from build123d import *

# Parameters (mm, degrees)
F0_R     = 75
F1_DEPTH = 3.5
F2_R     = 1.6
F3_DEPTH = 3.5
F5_DEPTH = 3.5
F6_R     = 1.6
F7_DEPTH = 3.5
F8_W     = 1.85
F8_H     = 28.2
F9_DEPTH = 3.501


with BuildPart() as f1:
    # F0 (on Top) → F1 (new body)
    with BuildSketch(Plane.XY):
        Circle(F0_R)
    extrude(amount=F1_DEPTH)

    # F2 (on Top) → F3 (cut)
    with BuildSketch(Plane.XY):
        with BuildLine():
            ThreePointArc((-35, -28.4), (-36.1313708499, -31.1313708499), (-33.4, -30))
            Line((-33.4, -30), (-35, -30))
            Line((-35, -30), (-35, -28.4))
        make_face()
        with BuildLine():
            Line((-35, -30), (-33.4, -30))
            ThreePointArc((-33.4, -30), (-33.8686291501, -28.8686291501), (-35, -28.4))
            Line((-35, -28.4), (-35, -30))
        make_face()
        with Locations((-50, 0)):
            Circle(F2_R)
        with BuildLine():
            ThreePointArc((51.6, 0), (50, 1.6), (48.4, 0))
            ThreePointArc((48.4, 0), (50, -1.6), (51.6, 0))
        make_face()
        with BuildLine():
            ThreePointArc((35, -28.4), (33.8686291501, -28.8686291501), (33.4, -30))
            Line((33.4, -30), (35, -30))
            Line((35, -30), (35, -28.4))
        make_face()
        with BuildLine():
            Line((35, -30), (33.4, -30))
            ThreePointArc((33.4, -30), (35, -31.6), (36.6, -30))
            ThreePointArc((36.6, -30), (36.1313708499, -28.8686291501), (35, -28.4))
            Line((35, -28.4), (35, -30))
        make_face()
        with BuildLine():
            ThreePointArc((-33.4, 30), (-36.1313708499, 31.1313708499), (-35, 28.4))
            Line((-35, 28.4), (-35, 30))
            Line((-35, 30), (-33.4, 30))
        make_face()
        with BuildLine():
            Line((-35, 30), (-35, 28.4))
            ThreePointArc((-35, 28.4), (-33.8686291501, 28.8686291501), (-33.4, 30))
            Line((-33.4, 30), (-35, 30))
        make_face()
        with BuildLine():
            ThreePointArc((-18.4, 0), (-20, 1.6), (-21.6, 0))
            Line((-21.6, 0), (-20, 0))
            Line((-20, 0), (-18.4, 0))
        make_face()
        with BuildLine():
            Line((-20, 0), (-21.6, 0))
            ThreePointArc((-21.6, 0), (-20, -1.6), (-18.4, 0))
            Line((-18.4, 0), (-20, 0))
        make_face()
        with BuildLine():
            ThreePointArc((33.4, 30), (33.8686291501, 28.8686291501), (35, 28.4))
            Line((35, 28.4), (35, 30))
            Line((35, 30), (33.4, 30))
        make_face()
        with BuildLine():
            Line((35, 30), (35, 28.4))
            ThreePointArc((35, 28.4), (36.1313708499, 28.8686291501), (36.6, 30))
            ThreePointArc((36.6, 30), (35, 31.6), (33.4, 30))
            Line((33.4, 30), (35, 30))
        make_face()
        with BuildLine():
            ThreePointArc((18.4, 0), (20, -1.6), (21.6, 0))
            Line((21.6, 0), (20, 0))
            Line((20, 0), (18.4, 0))
        make_face()
        with BuildLine():
            Line((20, 0), (21.6, 0))
            ThreePointArc((21.6, 0), (20, 1.6), (18.4, 0))
            Line((18.4, 0), (20, 0))
        make_face()
        with BuildLine():
            ThreePointArc((2.6, 0), (0, 2.6), (-2.6, 0))
            Line((-2.6, 0), (2.6, 0))
        make_face()
        with BuildLine():
            Line((2.6, 0), (-2.6, 0))
            ThreePointArc((-2.6, 0), (0, -2.6), (2.6, 0))
        make_face()
    extrude(amount=F3_DEPTH, mode=Mode.SUBTRACT)

    # F4 (on face) → F5 (join)
    with BuildSketch(Plane.XY.offset(3.5)):
        with BuildLine():
            ThreePointArc((29.5025076199, -68.9536224149), (40.7469515469, -74.139754822), (48.4136259754, -64.4157848623))
            ThreePointArc((48.4136259754, -64.4157848623), (47.9604080116, -61.4393855689), (46.6418354247, -58.732777801))
            ThreePointArc((46.6418354247, -58.732777801), (38.4136259754, -64.4157848623), (29.5025076199, -68.9536224149))
        make_face()
    extrude(amount=-F5_DEPTH)

    # F6 (on face) → F7 (cut)
    with BuildSketch(Plane.XY.offset(3.5)):
        with Locations((38.4136259754, -64.4157848623)):
            Circle(F6_R)
    extrude(amount=-F7_DEPTH, mode=Mode.SUBTRACT)

    # F8 (on face) → F9 (cut, through all)
    with BuildSketch(Plane.XY.offset(3.5)):
        with Locations((-34.075, 0)):
            Rectangle(F8_W, F8_H)
        with Locations((-35.925, 0)):
            Rectangle(F8_W, F8_H)
        with Locations((35.925, 0)):
            Rectangle(F8_W, F8_H)
        with Locations((34.075, 0)):
            Rectangle(F8_W, F8_H)
    extrude(amount=-F9_DEPTH, mode=Mode.SUBTRACT)


solid = f1.part
Input: part model. Units: mm. Frame: model coordinates. A direction names the side the tool comes from. Coordinates: 2 decimals unless noted, no trailing zeros. Loops run counter-clockwise (first coordinate to the right, second up) from the corner with the lowest first, then second, coordinate; pieces in that order, holes last. Notation, with made-up numbers: (-35.5, 76.5) - (-24.5, 76.5) arc R25 cw to (-24.5, 105.5) - close; hole circle Ø10 at (68.5, 56). An arc over 180 degrees is marked (long way). Answer in a Markdown table with one row per item. Add a question column.
Item 1: Line query: line 1 along X through (y, z) = (8.5, 1.95); line 2 along Y through (x, z) = (-35, 2.6); line 3 along Y through (x, z) = (0, 2). Output: solid intervals per line, ascending. Write a range as [from, to].
Item 2: Section query D-D on y = -45. Return the cut outline in (x, z), then the cut area to 3 significant figures.
Item 3: Access query for faces 3 (the flat face through (-35, -14.1, 2)), 4 (the flat face through (16, 1, 3.5)). Directions: +Z, -Z, +X, -X, +Y, -Y. A direction counts if a zero-diameter tool reaches every point of the face in a straight line with its end or side. Return the directions, or none.
Item 4: Section query A-A on x = 0. Return the cut outline in (y, z).
Item 5: Section query B-B on z = 2.4. State how many separate pieces and enclosed holes the cut face has, then the cut area to 3 significant figures.
Item 6: Mould query, pull axis Y, two halves, no side actions, for faces 1 (the cylindrical face through (-18.4, -0.07, 1.73)), 2 (the flat face through (16, 1, 0)). Classes: released by +Y, released by -Y, zero draft, split by the parting line, or undercut.
Item 7: Contact query for flat-ended pins moving along their axis: P1, Ø1, axis at y = 4, z = 2.5, coming from the +X side; P2, Ø1, axis at x = -35.5, z = 1, coming from the +Y side. Output: stop coordinate, or through.
Item 8: Section query C-C on y = -11. Return the cut outline in (x, z), then the cut area to 3 significant figures.
Recorded:
| question | item | result |
|---|---|---|
| 1 | line 1 | [-74.52, -36.85], [-33.15, 33.15], [36.85, 74.52] |
| 1 | line 2 | [-66.33, -31.6], [-28.4, -14.1], [14.1, 28.4], [31.6, 66.33] |
| 1 | line 3 | [-75, -2.6], [2.6, 75] |
| 2 | outline | (-60, 0) - (60, 0) - (60, 3.5) - (-60, 3.5) - close |
| 2 | area | 420 mm^2 |
| 3 | face 3 | +Z, -Z |
| 3 | face 4 | +Z, +X, -X, +Y, -Y |
| 4 | outline | (-75, 0) - (-2.6, 0) - (-2.6, 3.5) - (-75, 3.5) - close; (2.6, 0) - (75, 0) - (75, 3.5) - (2.6, 3.5) - close |
| 5 | separate pieces | 1 |
| 5 | enclosed holes | 12 |
| 5 | area | 17,500 mm^2 |
| 6 | face 1 | undercut |
| 6 | face 2 | zero draft |
| 7 | P1 | x = 74.92 |
| 7 | P2 | y = 66.33 |
| 8 | outline | (-74.19, 0) - (-36.85, 0) - (-36.85, 3.5) - (-74.19, 3.5) - close; (-33.15, 0) - (33.15, 0) - (33.15, 3.5) - (-33.15, 3.5) - close; (36.85, 0) - (74.19, 0) - (74.19, 3.5) - (36.85, 3.5) - close |
| 8 | area | 493 mm^2 |
